Autodesk Inventor part; units mm, degrees
ref_plane "YZ Plane" through (0, 0, 0) normal (1, 0, 0) x (0, 1, 0)
ref_plane "XZ Plane" through (0, 0, 0) normal (0, 1, 0) x (-1, 0, 0)
ref_plane "XY Plane" through (0, 0, 0) normal (0, 0, 1) x (1, 0, 0)
sketch "Sketch1" plane through (0, 0, 0) normal (0, 0, 1) x (1, 0, 0)
  line L0 (-84.455, 0) -> (84.455, 0)
  line L1 (0, -53.34) -> (0, 53.34)
  line L2 (60.325, 38.1) -> (60.325, -38.1)
  line L3 (-60.325, -38.1) -> (-60.325, 38.1)
  line L4 (44.45, 38.1) -> (44.45, -38.1) construction
  line L5 (-44.45, -38.1) -> (-44.45, 38.1) construction
  line L6 (-33.655, -27.305) -> (33.655, -27.305)
  line L7 (-44.45, 38.1) -> (-33.655, 27.305)
  line L8 (-60.325, 38.1) -> (-44.45, 38.1)
  line L9 (44.45, 38.1) -> (60.325, 38.1)
  line L10 (33.655, 27.305) -> (-33.655, 27.305)
  line L11 (33.655, 27.305) -> (44.45, 38.1)
  line L12 (-44.45, -38.1) -> (-33.655, -27.305)
  line L13 (44.45, -38.1) -> (33.655, -27.305)
  line L14 (60.325, -38.1) -> (44.45, -38.1)
  line L15 (-44.45, -38.1) -> (-60.325, -38.1)
  point P0 (0, 0)
  point P1 (-60.325, 0)
  point P2 (0, 27.305)
  dimension "d1" = 76.2
  dimension "d2" = 15.875
  dimension "d4" = 45
  dimension "d5" = 54.61
  dimension "d6" = 120.65
  dimension "d7" = 15.875
  dimension "d8" = 45
  dimension "d9" = 10.795
extrude "Extrusion1" add sketch "Sketch1" against normal blind 12.7
sketch "Sketch2" plane through (-33.655, 27.305, 0) normal (0, 1, 0) x (1, 0, 0)
  line L0 (67.31, 12.7) -> (0, 12.7)
  line L1 (67.31, 0) -> (67.31, 12.7)
  line L2 (0, 12.7) -> (-10.795, 12.7)
  line L3 (-10.795, 0) -> (-10.795, 12.7)
  line L4 (0, 0) -> (-10.795, 0)
  line L5 (0, 0) -> (0, 12.7)
  line L6 (-10.795, 12.7) -> (-26.67, 12.7)
  line L7 (-26.67, 0) -> (-26.67, 12.7)
  line L8 (-10.795, 0) -> (-26.67, 0)
  line L9 (-10.795, 0) -> (-10.795, 12.7)
  line L10 (-10.795, 12.7) -> (-26.67, 12.7)
  line L11 (-26.67, 0) -> (-26.67, 12.7)
  line L12 (-10.795, 0) -> (-10.795, 12.7)
  line L13 (93.98, 0) -> (78.105, 0)
  line L14 (78.105, 0) -> (67.31, 0)
  line L15 (78.105, 0) -> (78.105, 12.7)
  line L16 (78.105, 12.7) -> (67.31, 12.7)
  line L17 (93.98, 12.7) -> (78.105, 12.7)
  line L18 (93.98, 12.7) -> (78.105, 12.7)
  line L19 (78.105, 0) -> (78.105, 12.7)
  line L20 (93.98, 0) -> (78.105, 0)
  line L21 (93.98, 0) -> (93.98, 12.7)
  line L22 (33.655, 0) -> (33.655, 12.7) construction
  line L23 (59.055, 0) -> (59.055, 12.7) construction
  line L24 (8.255, 0.2933) -> (8.255, 12.9933) construction
  arc A0 (8.255, 7.0115) -> (59.055, 7.0115) centre (33.655, 60.325) ccw
  arc A1 (8.255, 12.7) -> (59.055, 12.7) centre (33.655, 60.325) ccw
  line L25 (66.421, 0.7551) -> (59.055, 7.0115)
  line L26 (59.055, 12.7) -> (67.31, 5.6885)
  line L27 (68.4764, 0) -> (93.98, 0)
  arc A2 (66.421, 0.7551) -> (68.4764, 0) centre (68.4764, 3.175) ccw
  line L28 (67.31, 5.6885) -> (93.98, 5.6885)
  line L29 (93.98, 0) -> (93.98, 5.6885)
  line L30 (0.889, 0.7551) -> (8.255, 7.0115)
  line L31 (8.255, 12.7) -> (0, 5.6885)
  line L32 (-1.1664, 0) -> (-26.67, 0)
  line L33 (0, 5.6885) -> (-26.67, 5.6885)
  line L34 (-26.67, 0) -> (-26.67, 5.6885)
  arc A3 (-1.1664, 0) -> (0.889, 0.7551) centre (-1.1664, 3.175) ccw
  dimension "d12" = 50.8
  dimension "d13" = 53.975
  dimension "d14" = 5.08
  dimension "d15" = 3.175
  dimension "d17" = 3.175
extrude "Extrusion2" cut sketch "Sketch2" along normal through all both and the other way through all contours L26 L1 A2 L25 A0 L30 A3 L5 L31 A1 | L28 L15 L14 A2 L1 | L28 L21 L13 L15 | L5 A3 L4 L3 L33 | L3 L8 L7 L33 keep common part
sketch "Sketch3" plane through (60.325, 38.1, -5.6885) normal (0, 0, -1) x (-1, 0, 0)
  line L0 (0, 0) -> (0, -76.2)
  line L1 (26.67, -65.405) -> (26.67, -10.795)
  line L2 (0, -38.1) -> (26.67, -38.1) construction
  point P0 (60.325, -38.1)
  point P1 (9.271, -9.525)
  point P2 (9.271, -66.675)
  dimension "d20" = 57.15
  dimension "d21" = 9.271
hole "Hole1" at (51.054, 28.575, -5.6885) at (51.054, -28.575, -5.6885) direction (0, 0, 1) diameter 8.89 end through all
mirror "Mirror1" about plane through (0, 0, 0) normal (1, 0, 0) of "Hole1"
equation "\"d9\" = -0.5 * d5 + 0.5 * d1"
properties part number "mount plate" material "Steel"
Verification items for the finished model (mm, model axes). A direction names the side the tool comes from. Give positions to 0.01 mm unless a question says otherwise; leave off trailing zeros. Loops run counter-clockwise (first coordinate to the right, second up) from the corner with the lowest first, then second, coordinate; pieces in that order, holes last.
1) Draft check along X on faces 5 (the flat face through (38.98, 32.63, -2.8)), 6 (the flat face through (47, -1, -5.688)), 7 (the flat face through (29.47, -0.382, -9.243)). Enter one of: pulls with the +X half, pulls with the -X half, needs draft (parallel to the pull), parting line crosses it, or undercut.
2) Depth check by flat-ended pin: pin 1 Ø8 at (x, y) = (42.5, 16) entering from -Z; pin 2 Ø10 at (x, y) = (13, -13) entering from +Z; pin 3 Ø4 at (x, y) = (-13.5, -24) entering from +Z. Enter the tip coordinate at first touch or a pass-through.
3) Set-up check for faces 1 (the flat face through (-47, -1, -5.688)), 2 (the flat face through (-29.135, -0.382, -3.84)), 3 (the flat face through (39.13, -32.78, -2.8)), 4 (the flat face through (0, 27.305, -5)): record each of +Z, -Z, +X, -X, +Y, -Y from which the full face is reachable in a straight line by a thin tool's end or side.
4) Sectioned sample at D-D, the plane x = 49. Enter the section's corners in (y, z).
5) Sectioned sample at C-C, the plane z = -3.25. Enter the section's corners in (x, y) (3 decimals), then the cut area to 3 significant figures.
6) Thickness scan on line 1 along Y through (x, z) = (-0.5, -3.5) (3 decimals); line 2 along Y through (x, z) = (-54.5, -4.5); line 3 along Z through (x, y) = (37.5, -24). Record the ranges inside material, lowest first.
7) Sectioned sample at A-A, the plane z = -10. Enter the section's corners in (x, y) (3 decimals), then the cut area to 3 significant figures.
Answers:
1. face 5: undercut
1. face 6: needs draft
1. face 7: pulls with the +X half
2. pin 1: stops at z = -5.69
2. pin 2: stops at z = -1.81
2. pin 3: stops at z = -2.4
3. face 1: -Z, -X, +Y, -Y
3. face 2: +Z, +Y, -Y
3. face 3: +Z, -Z, -Y
3. face 4: +Z, -Z, +Y
4. outline: (-38.1, -5.69) - (-32.52, -5.69) - (-32.52, 0) - (-38.1, 0) - close; (-24.63, -5.69) - (24.63, -5.69) - (24.63, 0) - (-24.63, 0) - close; (32.52, -5.69) - (38.1, -5.69) - (38.1, 0) - (32.52, 0) - close
5. outline: (-60.325, -38.1) - (-44.45, -38.1) - (-33.655, -27.305) - (-29.829, -27.305) - (-29.829, 27.305) - (-33.655, 27.305) - (-44.45, 38.1) - (-60.325, 38.1) - close; (-15.164, -27.305) - (15.164, -27.305) - (15.164, 27.305) - (-15.164, 27.305) - close; (29.829, -27.305) - (33.655, -27.305) - (44.45, -38.1) - (60.325, -38.1) - (60.325, 38.1) - (44.45, 38.1) - (33.655, 27.305) - (29.829, 27.305) - close; hole circle Ø8.89 at (-51.054, -28.575); hole circle Ø8.89 at (-51.054, 28.575); hole circle Ø8.89 at (51.054, -28.575); hole circle Ø8.89 at (51.054, 28.575)
5. area: 5,660 mm2
6. line 1: y = -27.305 to 27.305
6. line 2: y = -38.1 to -31.38, -25.77 to 25.77, 31.38 to 38.1
6. line 3: z = -5.69 to 0
7. outline: (-28.579, -27.305) - (-19.511, -27.305) - (-19.511, 27.305) - (-28.579, 27.305) - close; (19.511, -27.305) - (28.579, -27.305) - (28.579, 27.305) - (19.511, 27.305) - close
7. area: 990 mm2
